Verification items for the finished model (mm, model axes). A direction names the side the tool comes from. Round coordinates to 2 decimals unless told otherwise and drop trailing zeros. Write each loop counter-clockwise with the first axis right and the second up, starting at its lowest first coordinate (ties: lowest second). Pieces come first, ordered by that corner, then holes. Notation, with made-up numbers: (19, -7.5) -> (76, -7.5) arc R35 ccw to (76, 31.5) -> close; hole circle Ø9 at (-33, -34.5). An arc over 180 degrees is marked (long way). Answer as a JSON object with one key per item and string values. Group by question number.
(1) Sectioned sample at C-C on x = 26. Record the cut outline in (y, z).
(2) Set-up check for faces 1 (the face through (33, 3, 2)), 2 (the face through (55.014, 3.905, -0.867)): record each of +Z, -Z, +X, -X, +Y, -Y from which the full face is reachable in a straight line by a thin tool's end or side.
(3) Draft check along X on faces 3 (the face through (56, 0, 0)), 4 (the face through (18.703, 3.905, -0.867)), 5 (the face through (54, 3, -2)). Enter one of: released by +X, released by -X, zero draft, split by the parting line, or undercut.
(4) Gauge pin test, flat ends, axial feed: pin 1 Ø1 at (x, y) = (42.5, -1) entering from +Z; pin 2 Ø4 at (x, z) = (44, -3) entering from +Y; pin 3 Ø2.5 at (y, z) = (1.5, 1.5) entering from -X. Record the tip position at first contact, or that the pin passes through.
(5) Scan lines: L1, parallel to X at y = -3.5, z = -0.5; L2, parallel to Y at x = 25, z = 0.25; L3, parallel to X at y = 3.25, z = 1.75. Record each from-to range of solid material in increasing order. Write a range as from..to.
(6) Sectioned sample at A-A on y = 0. Record the cut outline in (x, z), and give its area (3 significant figures).
(7) Sectioned sample at D-D on x = 46.5. Record the cut outline in (y, z), and give its area (3 significant figures).
```python
from build123d import *

# Parameters (mm, degrees)
FILLET1_R = 4


with BuildPart() as part:
    # Sketch1 → Revolve1 (revolve)
    with BuildSketch(Plane.XY, mode=Mode.PRIVATE) as revolve1_sk:
        Polygon((0, 0), (0, 4), (33, 4), (33, 3.1), (54, 3.1), (54, 4), (56, 4), (56, 0), align=None)
    revolve(revolve1_sk.sketch.rotate(Axis((0, 0, 0), (1, 0, 0)), 90), axis=Axis((0, 0, 0), (1, 0, 0)))  # turned: the seam where the file's is

    # Fillet1
    fillet1_edges = [part.edges().sort_by_distance(p)[0] for p in [
        (0, 0, -4),
    ]]
    fillet(fillet1_edges, radius=FILLET1_R)


solid = part.part
```
Computed values:
{
 "1": {"outline": "circle Ø8 at (0, 0)"},
 "2": {"face 1": "none", "face 2": "+X, -X"},
 "3": {"face 3": "released by +X", "face 4": "zero draft", "face 5": "undercut"},
 "4": {"pin 1": "z = 3.06", "pin 2": "y = 2.93", "pin 3": "x = 0.1"},
 "5": {"L1": "2.13..33, 54..56", "L2": "-3.99..3.99", "L3": "2.46..33, 54..56"},
 "6": {"outline": "(4, -4) -> (33, -4) -> (33, -3.1) -> (54, -3.1) -> (54, -4) -> (56, -4) -> (56, 4) -> (54, 4) -> (54, 3.1) -> (33, 3.1) -> (33, 4) -> (4, 4) arc R4 ccw to start", "area": "403 mm2"},
 "7": {"outline": "circle Ø6.2 at (0, 0)", "area": "30.2 mm2"}
}
